Autodesk Inventor part; units mm, degrees
ref_plane "YZ Plane" through (0, 0, 0) normal (1, 0, 0) x (0, 1, 0)
ref_plane "XZ Plane" through (0, 0, 0) normal (0, 1, 0) x (-1, 0, 0)
ref_plane "XY Plane" through (0, 0, 0) normal (0, 0, 1) x (1, 0, 0)
sketch "스케치1" plane through (0, 0, 0) normal (0, 0, 1) x (1, 0, 0)
  line L0 (40, 40) -> (25, 40)
  line L1 (15, 40) -> (0, 40)
  line L2 (16, 40) -> (16, 35)
  line L3 (16, 35) -> (14, 35)
  line L4 (14, 35) -> (14, 36)
  line L5 (14, 36) -> (11, 36)
  line L6 (11, 36) -> (11, 31)
  line L7 (11, 31) -> (14, 28)
  line L8 (11, 31) -> (20.81, 31) construction
  line L9 (14, 28) -> (20, 28)
  line L10 (24, 40) -> (24, 35)
  line L11 (24, 35) -> (26, 35)
  line L12 (26, 35) -> (26, 36)
  line L13 (26, 36) -> (29, 36)
  line L14 (29, 36) -> (29, 31)
  line L15 (29, 31) -> (26, 28)
  line L16 (29, 31) -> (19.19, 31) construction
  line L17 (26, 28) -> (20, 28)
  line L18 (-0.0744, 15.9256) -> (4.9256, 15.9256)
  line L19 (-0.0744, 23.9256) -> (4.9256, 23.9256)
  line L20 (4.9256, 23.9256) -> (4.9256, 25.9256)
  line L21 (11.9256, 25.9256) -> (11.9256, 19.9256)
  line L22 (8.9256, 28.9256) -> (8.9256, 19.1155) construction
  line L23 (8.9256, 28.9256) -> (11.9256, 25.9256)
  line L24 (3.9256, 28.9256) -> (8.9256, 28.9256)
  line L25 (3.9256, 25.9256) -> (3.9256, 28.9256)
  line L26 (4.9256, 25.9256) -> (3.9256, 25.9256)
  line L27 (4.9256, 15.9256) -> (4.9256, 13.9256)
  line L28 (11.9256, 13.9256) -> (11.9256, 19.9256)
  line L29 (4.9256, 13.9256) -> (3.9256, 13.9256)
  line L30 (8.9256, 10.9256) -> (11.9256, 13.9256)
  line L31 (8.9256, 10.9256) -> (8.9256, 20.7356) construction
  line L32 (3.9256, 13.9256) -> (3.9256, 10.9256)
  line L33 (3.9256, 10.9256) -> (8.9256, 10.9256)
  line L34 (24, -0.1488) -> (24, 4.8512)
  line L35 (16, -0.1488) -> (16, 4.8512)
  line L36 (16, 4.8512) -> (14, 4.8512)
  line L37 (14, 11.8512) -> (20, 11.8512)
  line L38 (11, 8.8512) -> (20.81, 8.8512) construction
  line L39 (11, 8.8512) -> (14, 11.8512)
  line L40 (11, 3.8512) -> (11, 8.8512)
  line L41 (14, 3.8512) -> (11, 3.8512)
  line L42 (14, 4.8512) -> (14, 3.8512)
  line L43 (24, 4.8512) -> (26, 4.8512)
  line L44 (26, 11.8512) -> (20, 11.8512)
  line L45 (26, 4.8512) -> (26, 3.8512)
  line L46 (29, 8.8512) -> (26, 11.8512)
  line L47 (29, 8.8512) -> (19.19, 8.8512) construction
  line L48 (26, 3.8512) -> (29, 3.8512)
  line L49 (29, 3.8512) -> (29, 8.8512)
  line L50 (40.0744, 23.9256) -> (35.0744, 23.9256)
  line L51 (40.0744, 15.9256) -> (35.0744, 15.9256)
  line L52 (35.0744, 15.9256) -> (35.0744, 13.9256)
  line L53 (28.0744, 13.9256) -> (28.0744, 19.9256)
  line L54 (31.0744, 10.9256) -> (31.0744, 20.7356) construction
  line L55 (31.0744, 10.9256) -> (28.0744, 13.9256)
  line L56 (36.0744, 10.9256) -> (31.0744, 10.9256)
  line L57 (36.0744, 13.9256) -> (36.0744, 10.9256)
  line L58 (35.0744, 13.9256) -> (36.0744, 13.9256)
  line L59 (35.0744, 23.9256) -> (35.0744, 25.9256)
  line L60 (28.0744, 25.9256) -> (28.0744, 19.9256)
  line L61 (35.0744, 25.9256) -> (36.0744, 25.9256)
  line L62 (31.0744, 28.9256) -> (28.0744, 25.9256)
  line L63 (31.0744, 28.9256) -> (31.0744, 19.1155) construction
  line L64 (36.0744, 25.9256) -> (36.0744, 28.9256)
  line L65 (36.0744, 28.9256) -> (31.0744, 28.9256)
  line L66 (11, 20) -> (11.9256, 20)
  line L67 (28.0744, 20) -> (29, 20)
  line L68 (20, 3.8512) -> (20, 4.8512)
  line L69 (20, 35) -> (20, 36)
  line L70 (15, 40) -> (16, 40)
  line L71 (24, 40) -> (25, 40)
  line L72 (0, 40) -> (0, 23.9256)
  line L73 (0, 15.9256) -> (0, 0)
  line L74 (40, 0) -> (40, 15.9256)
  line L75 (40, 23.9256) -> (40, 40)
  line L76 (0, 0) -> (16, 0)
  line L77 (24, 0) -> (40, 0)
  point P0 (25, 38)
  point P1 (20, 19.9256)
  point P2 (15, 35)
  point P3 (25, 35)
  point P4 (4.9256, 24.9256)
  point P5 (4.9256, 14.9256)
  point P6 (15, 4.8512)
  point P7 (25, 4.8512)
  point P8 (35.0744, 14.9256)
  point P9 (35.0744, 24.9256)
  dimension "d0" = 40
  dimension "d1" = 40
  dimension "d14" = 2
  dimension "d15" = 5
  dimension "d16" = 1
  dimension "d17" = 3
  dimension "d18" = 5
  dimension "d19" = 45
  dimension "d21" = 7
  dimension "d24" = 360
extrude "돌출1" add sketch "스케치1" along normal mid plane 705
properties part number "70.5" material "철, 회색"
Geometry check sheet. Reference: the model listing, model coordinates, mm. A direction names the side the tool comes from. Round coordinates to 2 decimals unless told otherwise and drop trailing zeros. Write each question's results on one line, items separated by ' | '. Start each with the question number.
Q1. Gauge pin test, flat end, axial feed: P1, Ø2, axis at y = 8, z = -228.5, coming from the -X side. Record the tip position at first contact, or that the pin passes through.
Q2. Release check for a two-part mould opening along X. For faces 1 (the flat face through (40, 8, -5)), 2 (the flat face through (20, 11.851, -5)), 3 (the flat face through (20, 28, -5)), 4 (the flat face through (20, 20, -352.5)) record: +X half, -X half, draft (parallel to the pull), parting line (faces both ways), or undercut.
Q3. Access from +Z, -Z, +X, -X, +Y, -Y to the whole of each face (thin tool, end or side, straight path). Record for faces 5 (the flat face through (8, 0, -5)), 6 (the flat face through (11.926, 20, -5)).
Q4. Thickness scan on line 1 (Y direction, x = 24.5, z = -291); line 2 (X direction, y = 15, z = 53); line 3 (Y direction, x = 4, z = -226.5). Record the ranges inside material, lowest first. Write a range as [from, to].
Answers below:
1) P1: stops at x = 0
2) face 1: +X half | face 2: undercut | face 3: undercut | face 4: draft
3) face 5: +Z, -Z, +X, -X, -Y | face 6: +Z, -Z
4) line 1: y = [0, 4.85], [11.85, 28], [35, 40] | line 2: x = [0, 4.93], [11.93, 28.07], [35.07, 40] | line 3: y = [0, 10.93], [13.93, 15.93], [23.93, 25.93], [28.93, 40]
